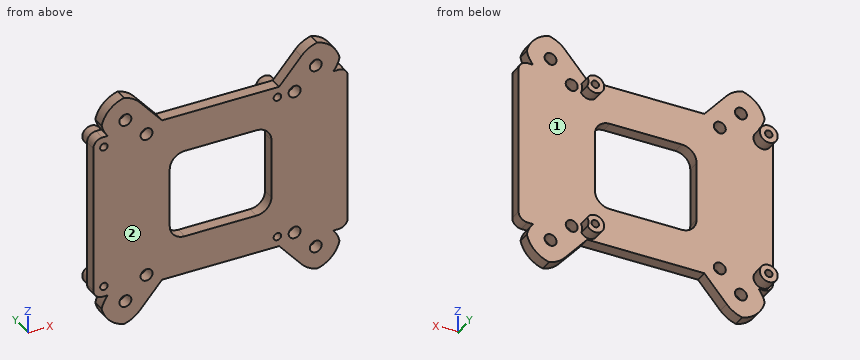
```python
from build123d import *

# Parameters (mm, degrees)
SKETCH1_W           = 85
SKETCH1_H           = 56
SKETCH1_R           = 1.25
BOSS_EXTRUDE1_DEPTH = 4
SKETCH2_R           = 3
SKETCH2_R_2         = 1.25
BOSS_EXTRUDE2_DEPTH = 4
FILLET1_R           = 3
BOSS_EXTRUDE4_DEPTH = 4
SKETCH3_R           = 2
CUT_EXTRUDE1_DEPTH  = 59.5
FILLET2_R           = 10
CUT_EXTRUDE2_START  = -10
SKETCH6_R           = 1.25
CUT_EXTRUDE2_DEPTH  = 10
SKETCH7_R           = 3.5
CUT_EXTRUDE3_DEPTH  = 10


with BuildPart() as part:
    # Sketch1 → Boss-Extrude1 (new body)
    with BuildSketch(Plane(origin=(0, 0, 0), x_dir=(1, 0, 0), z_dir=(0, 1, 0))):
        Rectangle(SKETCH1_W, SKETCH1_H)
        with Locations(Location((-39, 24.5, 0), (0, 0, 270))):
            Circle(SKETCH1_R, mode=Mode.SUBTRACT)
        with Locations(Location((-39, -24.5, 0), (0, 0, 270))):
            Circle(SKETCH1_R, mode=Mode.SUBTRACT)
        with Locations(Location((19, 24.5, 0), (0, 0, 270))):
            Circle(SKETCH1_R, mode=Mode.SUBTRACT)
        with Locations(Location((19, -24.5, 0), (0, 0, 270))):
            Circle(SKETCH1_R, mode=Mode.SUBTRACT)
        with BuildLine():
            Line((-12, -15), (12, -15))
            ThreePointArc((12, -15), (15.535533906, -13.535533906), (17, -10))
            Line((17, -10), (17, 10))
            ThreePointArc((17, 10), (15.535533906, 13.535533906), (12, 15))
            Line((12, 15), (-12, 15))
            ThreePointArc((-12, 15), (-15.535533906, 13.535533906), (-17, 10))
            Line((-17, 10), (-17, -10))
            ThreePointArc((-17, -10), (-15.535533906, -13.535533906), (-12, -15))
        make_face(mode=Mode.SUBTRACT)
    extrude(amount=BOSS_EXTRUDE1_DEPTH)

    # Sketch2 → Boss-Extrude2 (add)
    # profile 1 of 4: a face of its own
    with BuildSketch(Plane(origin=(0, 4, 0), x_dir=(1, 0, 0), z_dir=(0, 1, 0))):
        with Locations(Location((-39, 24.5, 0), (0, 0, 270))):
            Circle(SKETCH2_R)
        with Locations(Location((-39, 24.5, 0), (0, 0, 270))):
            Circle(SKETCH2_R_2, mode=Mode.SUBTRACT)
    # profile 2 of 4: a face of its own
    with BuildSketch(Plane(origin=(0, 4, 0), x_dir=(1, 0, 0), z_dir=(0, 1, 0))):
        with Locations(Location((19, 24.5, 0), (0, 0, 270))):
            Circle(SKETCH2_R)
        with Locations(Location((19, 24.5, 0), (0, 0, 270))):
            Circle(SKETCH2_R_2, mode=Mode.SUBTRACT)
    # profile 3 of 4: a face of its own
    with BuildSketch(Plane(origin=(0, 4, 0), x_dir=(1, 0, 0), z_dir=(0, 1, 0))):
        with Locations(Location((19, -24.5, 0), (0, 0, 270))):
            Circle(SKETCH2_R)
        with Locations(Location((19, -24.5, 0), (0, 0, 270))):
            Circle(SKETCH2_R_2, mode=Mode.SUBTRACT)
    # profile 4 of 4: a face of its own
    with BuildSketch(Plane(origin=(0, 4, 0), x_dir=(1, 0, 0), z_dir=(0, 1, 0))):
        with Locations(Location((-39, -24.5, 0), (0, 0, 270))):
            Circle(SKETCH2_R)
        with Locations(Location((-39, -24.5, 0), (0, 0, 270))):
            Circle(SKETCH2_R_2, mode=Mode.SUBTRACT)
    extrude(amount=BOSS_EXTRUDE2_DEPTH)

    # Fillet1
    fillet1_edges = [part.edges().sort_by_distance(p)[0] for p in [
        (-42.5, 2, 28),
        (-42.5, 2, -28),
        (42.5, 2, -28),
        (42.5, 2, 28),
    ]]
    fillet(fillet1_edges, radius=FILLET1_R)

    # Sketch5 → Boss-Extrude4 (add)
    with BuildSketch(Plane(origin=(0, 0, 0), x_dir=(1, 0, 0), z_dir=(0, 1, 0))):
        Polygon((-40, -30), (-17, -10), (-17, 10), (-40, 30), (-40, 40), (-30, 40), (-10, 17), (10, 17), (30, 40), (40, 40), (40, 30), (17, 10), (17, -10), (40, -30), (40, -40), (30, -40), (10, -17), (-10, -17), (-30, -40), (-40, -40), align=None)
    extrude(amount=BOSS_EXTRUDE4_DEPTH)

    # Sketch3 → Cut-Extrude1 (cut, through all)
    with BuildSketch(Plane(origin=(0, 4, 0), x_dir=(1, 0, 0), z_dir=(0, 1, 0))):
        with Locations(Location((-31.819805153, 31.819805153, 0), (0, 0, 270))):
            Circle(SKETCH3_R)
        with Locations(Location((-24.748737342, 24.748737342, 0), (0, 0, 270))):
            Circle(SKETCH3_R)
        with Locations(Location((31.819805153, 31.819805153, 0), (0, 0, 270))):
            Circle(SKETCH3_R)
        with Locations(Location((24.748737342, 24.748737342, 0), (0, 0, 270))):
            Circle(SKETCH3_R)
        with Locations(Location((24.748737342, -24.748737342, 0), (0, 0, 270))):
            Circle(SKETCH3_R)
        with Locations(Location((31.819805153, -31.819805153, 0), (0, 0, 270))):
            Circle(SKETCH3_R)
        with Locations(Location((-31.819805153, -31.819805153, 0), (0, 0, 270))):
            Circle(SKETCH3_R)
        with Locations(Location((-24.748737342, -24.748737342, 0), (0, 0, 270))):
            Circle(SKETCH3_R)
        with BuildLine():
            Line((12, -15), (-12, -15))
            ThreePointArc((-12, -15), (-15.535533906, -13.535533906), (-17, -10))
            Line((-17, -10), (-17, 10))
            ThreePointArc((-17, 10), (-15.535533906, 13.535533906), (-12, 15))
            Line((-12, 15), (12, 15))
            ThreePointArc((12, 15), (15.535533906, 13.535533906), (17, 10))
            Line((17, 10), (17, -10))
            ThreePointArc((17, -10), (15.535533906, -13.535533906), (12, -15))
        make_face()
    extrude(amount=-CUT_EXTRUDE1_DEPTH, mode=Mode.SUBTRACT)

    # Fillet2
    # the kernel refuses this fillet: 10 mm, written as the material it takes off along each edge
    with BuildSketch(Plane(origin=(-40, -10.951097141, -30), x_dir=(0.7546055221635131, 0, 0.6561787149247771), z_dir=(0, 1, 0))) as fillet2_piece_1_section:
        with BuildLine():
            CenterArc((4.671704482, 9.8672905), FILLET2_R, 221.009086902, 39.646111147)
            Line((-2.87435074, 3.305503351), (-3.025271844, 3.174267608))
            Line((-3.025271844, 3.174267608), (-0.150921104, -0.131235743))
            Line((-0.150921104, -0.131235743), (0, -0.2))
            ThreePointArc((0, -0.2), (1.523975065, -0.2), (3.015475044, -0.19734581))
            Line((3.015475044, -0.19734581), (3.047950131, 0))
        make_face()
    fillet2_piece_1 = extrude(amount=25.902194282, mode=Mode.PRIVATE)
    fillet2_piece_1 = split(fillet2_piece_1, bisect_by=Plane(origin=(-39.506364614, 2, -28), z_dir=(0, 0, -1)), keep=Keep.TOP, mode=Mode.PRIVATE)
    add(fillet2_piece_1, mode=Mode.SUBTRACT)
    with BuildSketch(Plane(origin=(-40, -25, -40), x_dir=(0, 0, 1), z_dir=(0, 1, 0)), Plane(origin=(40, -25, -40), x_dir=(-1, 0, 0), z_dir=(0, 1, 0))) as fillet2_piece_2:
        with BuildLine():
            CenterArc((FILLET2_R, FILLET2_R), FILLET2_R, 180, 90)
            Line((0, FILLET2_R), (-FILLET2_R * 0.02, FILLET2_R))
            Line((-FILLET2_R * 0.02, FILLET2_R), (-FILLET2_R * 0.02, -FILLET2_R * 0.02))
            Line((-FILLET2_R * 0.02, -FILLET2_R * 0.02), (FILLET2_R, -FILLET2_R * 0.02))
            Line((FILLET2_R, -FILLET2_R * 0.02), (FILLET2_R, 0))
        make_face()
    extrude(amount=54, mode=Mode.SUBTRACT)
    with BuildSketch(Plane(origin=(-30, -11.390762292, -40), x_dir=(-1, 0, 0), z_dir=(0, 1, 0)), Plane(origin=(30, -11.390762292, -40), x_dir=(-0.6561787149247741, 0, 0.7546055221635154), z_dir=(0, 1, 0))) as fillet2_piece_3:
        with BuildLine():
            CenterArc((FILLET2_R * 0.455630491663, FILLET2_R), FILLET2_R, 221.009086902, 48.990913098)
            Line((-FILLET2_R * 0.2989750305, FILLET2_R * 0.343821285075), (-FILLET2_R * 0.314067140943, FILLET2_R * 0.330697710777))
            Line((-FILLET2_R * 0.314067140943, FILLET2_R * 0.330697710777), (-FILLET2_R * 0.00911260983327, -FILLET2_R * 0.02))
            Line((-FILLET2_R * 0.00911260983327, -FILLET2_R * 0.02), (FILLET2_R * 0.455630491663, -FILLET2_R * 0.02))
            Line((FILLET2_R * 0.455630491663, -FILLET2_R * 0.02), (FILLET2_R * 0.455630491663, 0))
        make_face()
    extrude(amount=26.781524583, mode=Mode.SUBTRACT)
    with BuildSketch(Plane(origin=(40, -10.951097141, -30), x_dir=(0, 0, -1), z_dir=(0, 1, 0))) as fillet2_piece_4_section:
        with BuildLine():
            CenterArc((4.380438856, 10), FILLET2_R, 230.353888853, 39.646111147)
            Line((-2, 2.3), (-2.127608777, 2.146))
            ThreePointArc((-2.127608777, 2.146), (-1.150921104, 1.018764257), (-0.150921104, -0.131235743))
            Line((-0.150921104, -0.131235743), (0, -0.2))
            Line((0, -0.2), (4.380438856, -0.2))
            Line((4.380438856, -0.2), (4.380438856, 0))
        make_face()
    fillet2_piece_4 = extrude(amount=25.902194282, mode=Mode.PRIVATE)
    fillet2_piece_4 = split(fillet2_piece_4, bisect_by=Plane(origin=(39.506364614, 2, -28), z_dir=(0, 0, -1)), keep=Keep.TOP, mode=Mode.PRIVATE)
    add(fillet2_piece_4, mode=Mode.SUBTRACT)
    with BuildSketch(Plane(origin=(40, -10.951097141, 30), x_dir=(0, 0, 1), z_dir=(0, 1, 0))) as fillet2_piece_5_section:
        with BuildLine():
            CenterArc((4.380438856, -10), FILLET2_R, 90, 39.646111147)
            Line((-2, -2.3), (-2.127608777, -2.146))
            ThreePointArc((-2.127608777, -2.146), (-1.150921104, -1.018764257), (-0.150921104, 0.131235743))
            Line((-0.150921104, 0.131235743), (0, 0.2))
            Line((0, 0.2), (4.380438856, 0.2))
            Line((4.380438856, 0.2), (4.380438856, 0))
        make_face()
    fillet2_piece_5 = extrude(amount=25.902194282, mode=Mode.PRIVATE)
    fillet2_piece_5 = split(fillet2_piece_5, bisect_by=Plane(origin=(39.506364614, 2, 28), z_dir=(0, 0, 1)), keep=Keep.TOP, mode=Mode.PRIVATE)
    add(fillet2_piece_5, mode=Mode.SUBTRACT)
    with BuildSketch(Plane(origin=(40, -25, 40), x_dir=(-1, 0, 0), z_dir=(0, 1, 0)), Plane(origin=(-40, -25, 40), x_dir=(0, 0, -1), z_dir=(0, 1, 0))) as fillet2_piece_6:
        with BuildLine():
            CenterArc((FILLET2_R, -FILLET2_R), FILLET2_R, 90, 90)
            Line((0, -FILLET2_R), (-FILLET2_R * 0.02, -FILLET2_R))
            Line((-FILLET2_R * 0.02, -FILLET2_R), (-FILLET2_R * 0.02, FILLET2_R * 0.02))
            Line((-FILLET2_R * 0.02, FILLET2_R * 0.02), (FILLET2_R, FILLET2_R * 0.02))
            Line((FILLET2_R, FILLET2_R * 0.02), (FILLET2_R, 0))
        make_face()
    extrude(amount=54, mode=Mode.SUBTRACT)
    with BuildSketch(Plane(origin=(30, -11.390762292, 40), x_dir=(-0.6561787149247873, 0, -0.7546055221635042), z_dir=(0, 1, 0)), Plane(origin=(-30, -11.390762292, 40), x_dir=(-1, 0, 0), z_dir=(0, 1, 0))) as fillet2_piece_7:
        with BuildLine():
            CenterArc((FILLET2_R * 0.455630491663, -FILLET2_R), FILLET2_R, 90, 48.990913098)
            Line((-FILLET2_R * 0.2989750305, -FILLET2_R * 0.343821285075), (-FILLET2_R * 0.314067140943, -FILLET2_R * 0.330697710777))
            Line((-FILLET2_R * 0.314067140943, -FILLET2_R * 0.330697710777), (-FILLET2_R * 0.00911260983327, FILLET2_R * 0.02))
            Line((-FILLET2_R * 0.00911260983327, FILLET2_R * 0.02), (FILLET2_R * 0.455630491663, FILLET2_R * 0.02))
            Line((FILLET2_R * 0.455630491663, FILLET2_R * 0.02), (FILLET2_R * 0.455630491663, 0))
        make_face()
    extrude(amount=26.781524583, mode=Mode.SUBTRACT)
    with BuildSketch(Plane(origin=(-40, -10.951097141, 30), x_dir=(0.7546055221635047, 0, -0.6561787149247865), z_dir=(0, 1, 0))) as fillet2_piece_8_section:
        with BuildLine():
            CenterArc((4.671704482, -9.8672905), FILLET2_R, 99.344801951, 39.646111147)
            Line((-2.87435074, -3.305503351), (-3.025271844, -3.174267608))
            Line((-3.025271844, -3.174267608), (-0.150921104, 0.131235743))
            Line((-0.150921104, 0.131235743), (0, 0.2))
            ThreePointArc((0, 0.2), (1.523975065, 0.2), (3.015475044, 0.19734581))
            Line((3.015475044, 0.19734581), (3.047950131, 0))
        make_face()
    fillet2_piece_8 = extrude(amount=25.902194282, mode=Mode.PRIVATE)
    fillet2_piece_8 = split(fillet2_piece_8, bisect_by=Plane(origin=(-39.506364614, 2, 28), z_dir=(0, 0, 1)), keep=Keep.TOP, mode=Mode.PRIVATE)
    add(fillet2_piece_8, mode=Mode.SUBTRACT)

    # Sketch6 → Cut-Extrude2 (cut)
    with BuildSketch(Plane(origin=(0, 4, 0), x_dir=(1, 0, 0), z_dir=(0, 1, 0)).offset(CUT_EXTRUDE2_START)):
        with Locations(Location((19, -24.5, 0), (0, 0, 270))):
            Circle(SKETCH6_R)
        with Locations(Location((19, 24.5, 0), (0, 0, 270))):
            Circle(SKETCH6_R)
    extrude(amount=CUT_EXTRUDE2_DEPTH, mode=Mode.SUBTRACT)

    # Sketch7 → Cut-Extrude3 (cut)
    with BuildSketch(Plane(origin=(0, 4, 0), x_dir=(1, 0, 0), z_dir=(0, 1, 0))):
        with Locations((24.748737342, -24.748737342)):
            Circle(SKETCH7_R)
        with Locations((24.748737342, 24.748737342)):
            Circle(SKETCH7_R)
    extrude(amount=CUT_EXTRUDE3_DEPTH, mode=Mode.SUBTRACT)


solid = part.part
```
For this review, take the finished solid that the model builds, in its own axes (mm). Face numbers are marked on the shaded views. A direction names the side the tool comes from. Coordinates: 2 decimals unless noted, no trailing zeros. Write each loop counter-clockwise with the first axis right and the second up, starting at its lowest first coordinate (ties: lowest second). Pieces come first, ordered by that corner, then holes.
(1) Add section A-A on z = -6.5. Give the boundary of the cut face in (x, y).
(2) Add section C-C on y = 7. Give the boundary of the cut face in (x, z), then the cut area to 3 significant figures.
(3) Wall thickness on probe 1 along X at (y, z) = (6.75, 24.5); probe 2 along Z at (x, y) = (5.5, 1.5); probe 3 along X at (y, z) = (2.5, 25): over which ranges is each line inside the solid? List them lowest first.
(4) Add section B-B on x = -4.5. Give the boundary of the cut face in (y, z).
(5) Add section D-D on y = 2.5. Count the separate pieces of the cut face and the enclosed holes in it, then the cut area to 3 significant figures.
(6) Tool access review of the marked faces 1 and 2: name each direction out of +Z, -Z, +X, -X, +Y, -Y from which nothing blocks a thin tool from reaching the whole face with its end or side.
(7) For pin 1 Ø1.4 at (x, y) = (38.5, 3) entering from +Z; pin 2 Ø1.4 at (x, y) = (-39, 2.5) entering from +Z; pin 3 Ø2 at (x, y) = (-5, 2.5) entering from +Z, all flat-tipped, find the tip position at first contact; note any pin that passes through.
Answer sheet:
1. outline: (-42.5, 0) - (-17, 0) - (-17, 4) - (-42.5, 4) - close; (17, 0) - (42.5, 0) - (42.5, 4) - (17, 4) - close
2. outline: circle Ø6 at (-39, -24.5); circle Ø6 at (-39, 24.5); (21.53, -26.12) arc R3.5 cw to (21.66, -23.11) arc R3 ccw (long way) to start; (21.53, 26.12) arc R3 ccw (long way) to (21.66, 23.11) arc R3.5 cw to start; hole circle Ø2.5 at (-39, -24.5); hole circle Ø2.5 at (-39, 24.5); hole circle Ø2.5 at (19, -24.5); hole circle Ø2.5 at (19, 24.5)
2. area: 90.4 mm2
3. probe 1: x = -42 to -40.25, -37.75 to -36, 16 to 17.75, 20.25 to 21.26
3. probe 2: z = -28 to -15, 15 to 28
3. probe 3: x = -42.5 to -40.15, -37.85 to -26.73, -22.76 to 17.85, 20.15 to 22.76, 26.73 to 42.5
4. outline: (0, -28) - (4, -28) - (4, -15) - (0, -15) - close; (0, 15) - (4, 15) - (4, 28) - (0, 28) - close
5. separate pieces: 1
5. enclosed holes: 13
5. area: 4,250 mm2
6. face 1: +Y
6. face 2: +Z, -Z, +X, -X, -Y
7. pin 1: stops at z = 36.26
7. pin 2: stops at z = 35.58
7. pin 3: stops at z = 28
